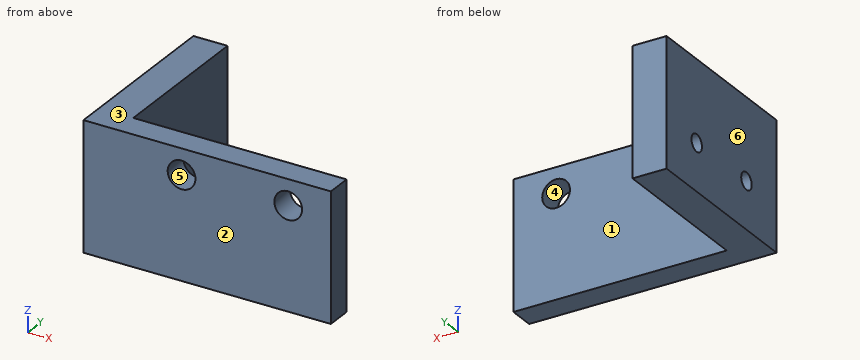
from build123d import *

# Parameters (mm, degrees)
SKETCH1_W           = 29
SKETCH1_H           = 15
BOSS_EXTRUDE1_DEPTH = 3
SKETCH3_R           = 1.625
CUT_EXTRUDE2_DEPTH  = 4
SKETCH4_W           = 4
SKETCH4_H           = 15
BOSS_EXTRUDE2_DEPTH = 18
SKETCH5_R           = 1
CUT_EXTRUDE3_DEPTH  = 13


with BuildPart() as part:
    # Sketch1 → Boss-Extrude1 (new body)
    with BuildSketch(Plane(origin=(0, 0, 0), x_dir=(1, 0, 0), z_dir=(0, 1, 0))):
        Rectangle(SKETCH1_W, SKETCH1_H)
    extrude(amount=BOSS_EXTRUDE1_DEPTH)

    # Sketch3 → Cut-Extrude2 (cut, through all)
    with BuildSketch(Plane(origin=(0, 3, 0), x_dir=(1, 0, 0), z_dir=(0, 1, 0))):
        with Locations((-3, -4.5)):
            Circle(SKETCH3_R)
        with Locations((9.5, -4.5)):
            Circle(SKETCH3_R)
    extrude(amount=-CUT_EXTRUDE2_DEPTH, mode=Mode.SUBTRACT)

    # Sketch4 → Boss-Extrude2 (add)
    with BuildSketch(Plane(origin=(0, 3, 0), x_dir=(1, 0, 0), z_dir=(0, 1, 0))):
        with Locations((-12.5, 0)):
            Rectangle(SKETCH4_W, SKETCH4_H)
    extrude(amount=BOSS_EXTRUDE2_DEPTH)

    # Sketch5 → Cut-Extrude3 (cut)
    with BuildSketch(Plane.ZY.offset(14.5)):
        with Locations((-2, 15.25)):
            Circle(SKETCH5_R)
        with Locations((-2, 5.75)):
            Circle(SKETCH5_R)
    extrude(amount=-CUT_EXTRUDE3_DEPTH, mode=Mode.SUBTRACT)


solid = part.part
The listing builds one solid part. Answer for the finished solid, in the listing's coordinates (mm). Face numbers are marked on the shaded views. A direction names the side the tool comes from. Give positions to 0.01 mm unless a question says otherwise; leave off trailing zeros. Loops run counter-clockwise (first coordinate to the right, second up) from the corner with the lowest first, then second, coordinate; pieces in that order, holes last.
Item 1: A cutting plane is placed at C-C (y = 15.25). Give the vertices of the cut face in (x, z), then the cut area to 3 significant figures.
Derived:
outline: (-14.5, -7.5) - (-10.5, -7.5) - (-10.5, -3) - (-14.5, -3) - close; (-14.5, -1) - (-10.5, -1) - (-10.5, 7.5) - (-14.5, 7.5) - close
area: 52.0 mm2
Item 2: A cutting plane is placed at A-A (x = 9.5). Give the vertices of the cut face in (y, z) (3 decimals), then the cut area to 4 significant figures.
Derived:
outline: (0, -7.5) - (3, -7.5) - (3, 2.875) - (0, 2.875) - close; (0, 6.125) - (3, 6.125) - (3, 7.5) - (0, 7.5) - close
area: 35.25 mm2
Item 3: A tool of negligible diameter and unlimited length cuts with its end or side. For the marked faces 1 and 2, from which of +Z, -Z, +X, -X, +Y, -Y can it reach the whole face along a straight path? Write none if from no direction.
Derived:
face 1: +Z, -Z, +X, +Y
face 2: +Z, -Z, +X, -X, -Y
Item 4: Each of these flat-tipped pins is pushed along its axis until it touches: pin 1 Ø7.5 at (x, z) = (5.5, -1) entering from +Y; pin 2 Ø1.9 at (x, z) = (9.5, 4.5) entering from -Y; pin 3 Ø2.5 at (y, z) = (5.75, -2) entering from +X. Where does it stop, or does it pass through?
Derived:
pin 1: stops at y = 3
pin 2: passes through
pin 3: stops at x = -10.5
Item 5: Find the intervals of material crossed by line 1 along Y through (x, z) = (-11.4, -2); line 2 along X through (y, z) = (2.35, 4.5) (3 decimals); line 3 along X through (y, z) = (17, -5.75), in increasing order.
Derived:
line 1: y = 0 to 4.75, 6.75 to 14.25, 16.25 to 21
line 2: x = -14.5 to -4.625, -1.375 to 7.875, 11.125 to 14.5
line 3: x = -14.5 to -10.5
Item 6: A cutting plane is placed at B-B (z = -2). Give the vertices of the cut face in (x, y).
Derived:
outline: (-14.5, 0) - (14.5, 0) - (14.5, 3) - (-10.5, 3) - (-10.5, 4.75) - (-14.5, 4.75) - close; (-14.5, 6.75) - (-10.5, 6.75) - (-10.5, 14.25) - (-14.5, 14.25) - close; (-14.5, 16.25) - (-10.5, 16.25) - (-10.5, 21) - (-14.5, 21) - close
Item 7: Determine the mould class of the marked faces 3, 4, 5 and 6 for opening direction X: +X half, -X half, draft (parallel to the pull), parting line (faces both ways), or undercut.
Derived:
face 3: draft
face 4: undercut
face 5: undercut
face 6: -X half
Item 8: A cutting plane is placed at D-D (z = 4.5). Give the vertices of the cut face in (x, y) (3 decimals), then the cut area to 4 significant figures.
Derived:
outline: (-14.5, 0) - (-4.625, 0) - (-4.625, 3) - (-10.5, 3) - (-10.5, 21) - (-14.5, 21) - close; (-1.375, 0) - (7.875, 0) - (7.875, 3) - (-1.375, 3) - close; (11.125, 0) - (14.5, 0) - (14.5, 3) - (11.125, 3) - close
area: 139.5 mm2
